CAD build for the part. Positions are in the model's coordinates, mm. A direction names the side the tool comes from. Give positions to 0.01 mm unless a question says otherwise; leave off trailing zeros. Order: outer loops, then holes, each group sorted by start corner. A loop starts at its lowest first (then second) coordinate and runs counter-clockwise, first axis right, second up.
Item 1: Band-saw the part on B-B on x = 4. Give the cut face in (y, z).
Item 2: Wall check: L1, parallel to X at y = -1, z = 2; L2, parallel to X at y = 3, z = 4; L3, parallel to Y at x = 5, z = 5.25. Give the ranges that are in metal, low to high.
Item 3: Band-saw the part on D-D on x = 14.5. Give the cut face in (y, z), plus the area to 3 significant figures.
Item 4: Band-saw the part on C-C on z = 3.5. Give the cut face in (x, y).
Item 5: Two-plate mould, pull along Y, no slides. Class faces 1 (the flat face through (10, 10.2, 3)), 2 (the cylindrical face through (13.579, 3.745, 3.245)), 3 (the flat face through (18.2, -2, 3)): released by +Y, released by -Y, zero draft, split by the parting line, or undercut.
Item 6: Which spindle directions (+Z, -Z, +X, -X, +Y, -Y) get a long thin tool onto all of the face, cutting with end or side? Do faces 4 (the flat face through (10, 5, 0)), 5 (the cylindrical face through (6.19, 3.28, 3.24)), 6 (the flat face through (18.6, -2, 3)), 7 (the flat face through (9.8, -2, 3)), 8 (the flat face through (2.1, -2, 3)). Say none if no direction does.
Item 7: Band-saw the part on A-A on y = 2.9. Give the cut face in (x, z).
Item 8: Flat gauge pins, fed straight in: P1, Ø1.6, axis at y = -1, z = 3, coming from the -X side; P2, Ø1, axis at y = -1.5, z = 3.5, coming from the +X side. Where does each tip first touch, or does it go through?
```python
from build123d import *

# Parameters (mm, degrees)
SKETCH1_W           = 20
SKETCH1_H           = 10.2
BOSS_EXTRUDE1_DEPTH = 6.4
SKETCH2_W           = 0.4
SKETCH2_H           = 3.3
BOSS_EXTRUDE2_DEPTH = 3.5
CUT_EXTRUDE1_REACH  = 8.4
SKETCH3_R           = 1.25
CHAMFER1_SIZE       = 0.5


with BuildPart() as part:
    # Sketch1 → Boss-Extrude1 (new body)
    with BuildSketch(Plane.XY):
        with Locations((10, 5.1)):
            Rectangle(SKETCH1_W, SKETCH1_H)
    extrude(amount=BOSS_EXTRUDE1_DEPTH)

    # Sketch2 → Boss-Extrude2 (add)
    with BuildSketch(Plane.XZ):
        with Locations((18.4, 3.2)):
            Rectangle(SKETCH2_W, SKETCH2_H)
        with Locations((9.6, 3.2)):
            Rectangle(SKETCH2_W, SKETCH2_H)
        with Locations((2.3, 3.2)):
            Rectangle(SKETCH2_W, SKETCH2_H)
    extrude(amount=BOSS_EXTRUDE2_DEPTH)

    # Sketch3 → Cut-Extrude1 (cut, up to next)
    with BuildSketch(Plane.XY.offset(6.4), mode=Mode.PRIVATE) as cut_extrude1_sk1:
        with Locations((14.5, 2.9)):
            Circle(SKETCH3_R)
    cut_extrude1_tool1 = extrude(cut_extrude1_sk1.sketch, amount=-CUT_EXTRUDE1_REACH, mode=Mode.PRIVATE) & part.part
    add(cut_extrude1_tool1.solids().sort_by_distance((14.5, 2.9, 6.4))[0], mode=Mode.SUBTRACT)
    # Sketch3 → Cut-Extrude1 (cut, up to next)
    with BuildSketch(Plane.XY.offset(6.4), mode=Mode.PRIVATE) as cut_extrude1_sk2:
        with Locations((5, 2.9)):
            Circle(SKETCH3_R)
    cut_extrude1_tool2 = extrude(cut_extrude1_sk2.sketch, amount=-CUT_EXTRUDE1_REACH, mode=Mode.PRIVATE) & part.part
    add(cut_extrude1_tool2.solids().sort_by_distance((5, 2.9, 6.4))[0], mode=Mode.SUBTRACT)

    # Chamfer1
    chamfer1_edges = [part.edges().sort_by_distance(p)[0] for p in [
        (18.4, -3.5, 1.55),
        (18.4, -3.5, 4.85),
        (9.6, -3.5, 1.55),
        (9.6, -3.5, 4.85),
        (2.3, -3.5, 1.55),
        (2.3, -3.5, 4.85),
    ]]
    chamfer(chamfer1_edges, length=CHAMFER1_SIZE)


solid = part.part
```
The answers:
1. outline: (0, 0) - (2.15, 0) - (2.15, 6.4) - (0, 6.4) - close; (3.65, 0) - (10.2, 0) - (10.2, 6.4) - (3.65, 6.4) - close
2. L1: x = 2.1 to 2.5, 9.4 to 9.8, 18.2 to 18.6
2. L2: x = 0 to 3.75, 6.25 to 13.25, 15.75 to 20
2. L3: y = 0 to 1.65, 4.15 to 10.2
3. outline: (0, 0) - (1.65, 0) - (1.65, 6.4) - (0, 6.4) - close; (4.15, 0) - (10.2, 0) - (10.2, 6.4) - (4.15, 6.4) - close
3. area: 49.3 mm2
4. outline: (0, 0) - (2.1, 0) - (2.1, -3.5) - (2.5, -3.5) - (2.5, 0) - (9.4, 0) - (9.4, -3.5) - (9.8, -3.5) - (9.8, 0) - (18.2, 0) - (18.2, -3.5) - (18.6, -3.5) - (18.6, 0) - (20, 0) - (20, 10.2) - (0, 10.2) - close; hole circle Ø2.5 at (5, 2.9); hole circle Ø2.5 at (14.5, 2.9)
5. face 1: released by +Y
5. face 2: undercut
5. face 3: zero draft
6. face 4: -Z, +X, -X, +Y, -Y
6. face 5: +Z, -Z
6. face 6: +Z, -Z, +X, -Y
6. face 7: +Z, -Z, -Y
6. face 8: +Z, -Z, -X, -Y
7. outline: (0, 0) - (3.75, 0) - (3.75, 6.4) - (0, 6.4) - close; (6.25, 0) - (13.25, 0) - (13.25, 6.4) - (6.25, 6.4) - close; (15.75, 0) - (20, 0) - (20, 6.4) - (15.75, 6.4) - close
8. P1: stops at x = 2.1
8. P2: stops at x = 18.6
